Could you check a few things on this model? Use its own coordinates, in mm. Coordinates: 2 decimals unless noted, no trailing zeros. Order: outer loops, then holes, each group sorted by start corner. A loop starts at its lowest first (then second) coordinate and runs counter-clockwise, first axis right, second up. Notation, with made-up numbers: (-27.75, 25) -> (-19.75, 25) arc R17 cw to (-19.75, 38) -> close; hole circle Ø8 at (4.25, 22). An arc over 180 degrees is marked (long way). Put each result on its own line as item: value. Start each with the question number.
Q1. Please list where these lines run through material, in increasing order: line 1 along X through (y, z) = (-1, 109.5); line 2 along Y through (x, z) = (0, 344); line 3 along Z through (x, y) = (-4, -2.5).
Q2. If we section it at A-A (x = 0): Please give me the cut outline in (y, z).
Q3. Will these pins go through, and if not, where does the flat tip stop? pin 1 (5 mm diameter, centred on y = -3.5, z = 515, fed in from +X); pin 2 (1.5 mm diameter, centred on x = -3.5, z = 270.5, fed in from -Y); pin 3 (1 mm diameter, centred on x = -3.5, z = 350, fed in from +Y).
Q4. If we section it at C-C (z = 513.5): Please give me the cut outline in (x, y), and give its area (3 significant figures).
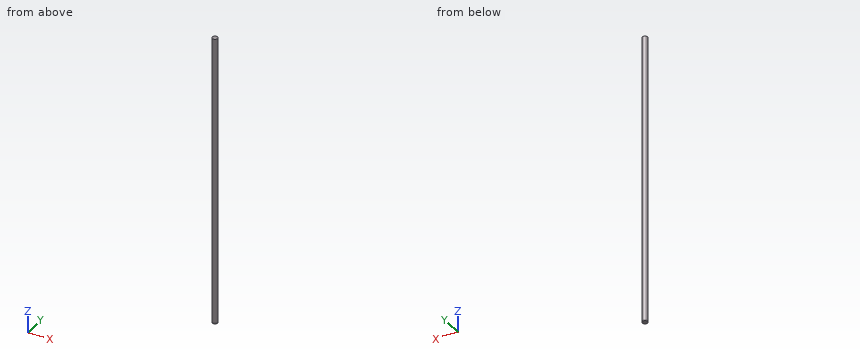
Autodesk Inventor part; units mm, degrees
ref_plane "YZ Plane" through (0, 0, 0) normal (1, 0, 0) x (0, 1, 0)
ref_plane "XZ Plane" through (0, 0, 0) normal (0, 1, 0) x (-1, 0, 0)
ref_plane "XY Plane" through (0, 0, 0) normal (0, 0, 1) x (1, 0, 0)
sketch "Sketch1" plane through (0, 0, 0) normal (0, 0, 1) x (1, 0, 0)
  circle A0 centre (0, 0) radius 7
  circle A1 centre (0, 0) radius 5
  dimension "d0" = 14
  dimension "d1" = 10
extrude "Extrusion1" add sketch "Sketch1" along normal blind 760
sketch "Sketch2" plane through (0, 0, 760) normal (0, 0, 1) x (1, 0, 0)
  circle A0 centre (0, 0) radius 7
extrude "Extrusion2" add sketch "Sketch2" along normal blind 2
sketch "Sketch3" plane through (0, 0, 0) normal (0, 0, -1) x (-1, 0, 0)
  circle A0 centre (0, 0) radius 7
extrude "Extrusion3" add sketch "Sketch3" along normal blind 2
properties part number "cięgno fotela"
The answers:
1. line 1: -6.93 to -4.9, 4.9 to 6.93
1. line 2: -7 to -5, 5 to 7
1. line 3: -2 to 0, 760 to 762
2. outline: (-7, -2) -> (7, -2) -> (7, 762) -> (-7, 762) -> close; hole (-5, 0) -> (5, 0) -> (5, 760) -> (-5, 760) -> close
3. pin 1: x = 6.93
3. pin 2: y = -6.44
3. pin 3: y = 6.32
4. outline: circle Ø14 at (0, 0); hole circle Ø10 at (0, 0)
4. area: 75.4 mm^2
